```python
from build123d import *

# Parameters (mm, degrees)
CHAMFER_1_SIZE = 0.5
CHAMFER_2_SIZE = 0.2


with BuildPart() as part:
    # Эскиз1 → Повернуть1 (revolve)
    with BuildSketch(Plane.XY, mode=Mode.PRIVATE) as revolve_1_sk:
        with BuildLine():
            Line((0.829156198, 14), (3.5, 14))
            Line((3.5, 14), (3.5, 12.5))
            Line((3.5, 12.5), (-3.5, 12.5))
            Line((-3.5, 12.5), (-3.5, 14))
            Line((-3.5, 14), (-0.829156198, 14))
            ThreePointArc((-0.829156198, 14), (0, 13.75), (0.829156198, 14))
        make_face()
    revolve(revolve_1_sk.sketch.rotate(Axis((0, 0, 0), (1, 0, 0)), 90), axis=Axis((0, 0, 0), (1, 0, 0)))

    # Фаска1
    chamfer_1_edges = [part.edges().sort_by_distance(p)[0] for p in [
        (3.5, 0, -12.5),
        (-3.5, 0, -12.5),
    ]]
    chamfer(chamfer_1_edges, length=CHAMFER_1_SIZE)

    # Фаска2
    chamfer_2_edges = [part.edges().sort_by_distance(p)[0] for p in [
        (-3.5, 0, -14),
        (3.5, 0, -14),
    ]]
    chamfer(chamfer_2_edges, length=CHAMFER_2_SIZE)


solid = part.part
```
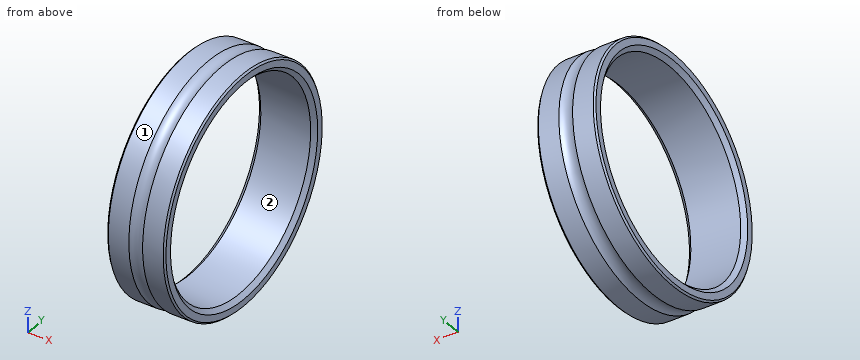
Build history of the part. All positions in model axes, mm. Face numbers are marked on the shaded views. Round coordinates to 2 decimals unless told otherwise and drop trailing zeros. Loops run counter-clockwise (first coordinate to the right, second up) from the corner with the lowest first, then second, coordinate; pieces in that order, holes last.
Item 1: Two-plate mould, pull along Y, no slides. Class the marked faces 1 and 2: released by +Y, released by -Y, zero draft, split by the parting line, or undercut.
Item 2: Saw through at A-A (y = 0). List the corners of the cut face in (x, z).
Item 3: Drill centre lines: line 1 along Y through (x, z) = (1.8, 0); line 2 along Y through (x, z) = (2.75, 5.25); line 3 along Z through (x, y) = (-2.75, -5.5). Where is each one in solid material? Low to high.
Item 4: Saw through at C-C (x = 1.5). List the corners of the cut face in (y, z).
Item 5: Pin check, flat tips, straight feed: P1, Ø4, axis at x = 0, y = 9, coming from the +Z side; P2, Ø2, axis at x = 1.5, y = 3, coming from the -Z side; P3, Ø8, axis at y = -10.5, z = 1.5, coming from the +X side. Stop position of each tip, or through.
Worked answers:
1. face 1: split by the parting line
1. face 2: undercut
2. outline: (-3.5, -13.8) - (-3.3, -14) - (-0.83, -14) arc R1.5 cw to (0.83, -14) - (3.3, -14) - (3.5, -13.8) - (3.5, -13) - (3, -12.5) - (-3, -12.5) - (-3.5, -13) - close; (-3.5, 13) - (-3, 12.5) - (3, 12.5) - (3.5, 13) - (3.5, 13.8) - (3.3, 14) - (0.83, 14) arc R1.5 cw to (-0.83, 14) - (-3.3, 14) - (-3.5, 13.8) - close
3. line 1: y = -14 to -12.5, 12.5 to 14
3. line 2: y = -12.98 to -11.34, 11.34 to 12.98
3. line 3: z = -12.87 to -11.22, 11.22 to 12.87
4. outline: circle Ø28 at (0, 0); hole circle Ø25 at (0, 0)
5. P1: stops at z = 12.02
5. P2: stops at z = -13.86
5. P3: stops at x = 3.5
